```python
from build123d import *

# Parameters (mm, degrees)
SKETCH2_W           = 35
SKETCH2_H           = 35
SKETCH2_R           = 1.6
BOSS_EXTRUDE1_DEPTH = 5
BOSS_EXTRUDE2_DEPTH = 2
SKETCH4_R           = 1.55
BOSS_EXTRUDE3_DEPTH = 2
CUT_EXTRUDE1_DEPTH  = 52.27194652
FILLET1_R           = 2


with BuildPart() as part:
    # Sketch2 → Boss-Extrude1 (new body)
    with BuildSketch(Plane(origin=(0, 0, 0), x_dir=(1, 0, 0), z_dir=(0, 1, 0))):
        Rectangle(SKETCH2_W, SKETCH2_H)
        with Locations(Location((7, 0, 0), (0, 0, 270))):
            Circle(SKETCH2_R, mode=Mode.SUBTRACT)
        with Locations(Location((-3.5, -6.062177826, 0), (0, 0, 270))):
            Circle(SKETCH2_R, mode=Mode.SUBTRACT)
        with Locations(Location((-3.5, 6.062177826, 0), (0, 0, 270))):
            Circle(SKETCH2_R, mode=Mode.SUBTRACT)
    extrude(amount=BOSS_EXTRUDE1_DEPTH)

    # Sketch3 → Boss-Extrude2 (add)
    with BuildSketch(Plane(origin=(17.5, 0, 0), x_dir=(0, 0, -1), z_dir=(1, 0, 0))):
        Polygon((-17.5, 0), (-27.5, 18.75), (17.5, 18.75), (17.5, 0), align=None)
    boss_extrude2 = extrude(amount=BOSS_EXTRUDE2_DEPTH)

    # Mirror1: Boss-Extrude2 across plane
    add(boss_extrude2.mirror(Plane(origin=(0, 0, 0), x_dir=(0, 0, 1), z_dir=(1, 0, 0))))

    # Sketch4 → Boss-Extrude3 (add)
    with BuildSketch(Plane(origin=(0, 18.75, 0), x_dir=(1, 0, 0), z_dir=(0, 1, 0))):
        Polygon((-19.5, -27.5), (-29.5, -27.5), (-19.5, 17.5), align=None)
        with Locations(Location((-23, -22.5, 0), (0, 0, 270))):
            Circle(SKETCH4_R, mode=Mode.SUBTRACT)
        with Locations(Location((-23, -10, 0), (0, 0, 270))):
            Circle(SKETCH4_R, mode=Mode.SUBTRACT)
    boss_extrude3 = extrude(amount=-BOSS_EXTRUDE3_DEPTH)

    # Sketch5 → Cut-Extrude1 (cut, through all)
    with BuildSketch(Plane(origin=(-19.5, 0, 0), x_dir=(0, 0, -1), z_dir=(1, 0, 0))):
        Polygon((-27.5, 18.75), (-26.433333333, 16.75), (-27.5, 16.75), align=None)
    cut_extrude1 = extrude(amount=-CUT_EXTRUDE1_DEPTH, mode=Mode.SUBTRACT)

    # Mirror2: Boss-Extrude3, Cut-Extrude1 across plane
    add(boss_extrude3.mirror(Plane(origin=(0, 0, 0), x_dir=(0, 0, 1), z_dir=(1, 0, 0))))
    add(cut_extrude1.mirror(Plane(origin=(0, 0, 0), x_dir=(0, 0, 1), z_dir=(1, 0, 0))), mode=Mode.SUBTRACT)

    # Fillet1
    fillet1_edges = [part.edges().sort_by_distance(p)[0] for p in [
        (17.5, 11.875, -17.5),
        (-17.5, 11.875, -17.5),
        (-17.5, 18.75, 5),
        (17.5, 18.75, 5),
        (0, 5, -17.5),
        (0, 0, -17.5),
        (17.5, 5, 0),
        (-17.5, 5, 0),
        (-19.5, 0, 0),
        (19.5, 0, 0),
    ]]
    fillet(fillet1_edges, radius=FILLET1_R - 0.0001)  # a hair under: the kernel refuses the full size


solid = part.part
```
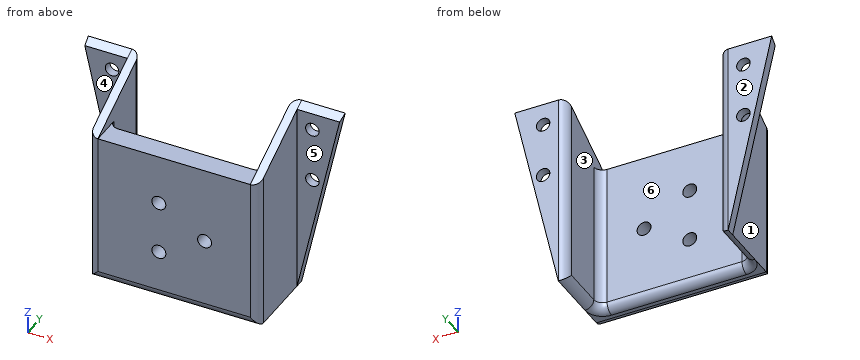
CAD build for the part. Positions are in the model's coordinates, mm. Face numbers are marked on the shaded views. A direction names the side the tool comes from. Round coordinates to 2 decimals unless told otherwise and drop trailing zeros. Order: outer loops, then holes, each group sorted by start corner. A loop starts at its lowest first (then second) coordinate and runs counter-clockwise, first axis right, second up. Notation, with made-up numbers: (47, 3) - (87, 3) arc R10 ccw to (87, 16) - close; hole circle Ø2 at (58, 83). An arc over 180 degrees is marked (long way). Answer as CSV lines item,"result". Start each with the question number.
1. Saw through at B-B, the plane x = -3.5. Write the cut outline in (y, z).
2. Saw through at A-A, the plane x = 7. Write the cut outline in (y, z).
3. Drill centre lines: L1, parallel to X at y = 15.25, z = 23.5; L2, parallel to X at y = 17.6, z = 10; L3, parallel to X at y = 18.2, z = 10. Where is each one in solid material? Low to high. Write a range as [from, to].
4. Pin check, flat tips, straight feed: pin 1 (1.5 mm diameter, centred on y = 5.5, z = 19, fed in from +X); pin 2 (4 mm diameter, centred on x = 8, z = 17.5, fed in from -Y); pin 3 (6 mm diameter, centred on x = 5, z = 9.5, fed in from +Y); pin 4 (5 mm diameter, centred on y = 10.5, z = 7, fed in from -X). Stop position of each tip, or through.
5. Tool access for the marked faces 4, 5 and 6: list every direction of +Z, -Z, +X, -X, +Y, -Y with a clear straight run to the whole face (end or side of a thin tool).
6. Pull direction X, two halves, no side cores. Call the marked faces 1, 2 and 3: +X half, -X half, draft (parallel to the pull), parting line (faces both ways), or undercut.
7. Saw through at C-C, the plane z = 0. Write the cut outline in (x, y), and give its area (3 significant figures).
Model answer:
1,outline,"(0, -15.5) arc R2 ccw to (2, -17.5) - (3, -17.5) arc R2 ccw to (5, -15.5) - (5, -7.66) - (0, -7.66) - close; (0, -4.46) - (5, -4.46) - (5, 4.46) - (0, 4.46) - close; (0, 7.66) - (5, 7.66) - (5, 17.5) - (0, 17.5) - close"
2,outline,"(0, -15.5) arc R2 ccw to (2, -17.5) - (3, -17.5) arc R2 ccw to (5, -15.5) - (5, -1.6) - (0, -1.6) - close; (0, 1.6) - (5, 1.6) - (5, 17.5) - (0, 17.5) - close"
3,L1,"x = [-19.5, -17.5], [17.5, 19.5]"
3,L2,"x = [-25.61, -24.55], [-21.45, -17.69], [17.69, 21.45], [24.55, 25.61]"
3,L3,"x = [-25.61, -24.55], [-21.45, -18.12], [18.12, 21.45], [24.55, 25.61]"
4,pin 1,"stops at x = 19.5"
4,pin 2,"stops at y = 0"
4,pin 3,"stops at y = 5"
4,pin 4,"stops at x = -19.5"
5,face 4,"+Z, -Z, -X, -Y"
5,face 5,"+Z, -Z, +X, -Y"
5,face 6,"+Z, -Z, +Y"
6,face 1,"-X half"
6,face 2,"draft"
6,face 3,"undercut"
7,outline,"(-23.39, 16.75) - (-19.5, 16.75) - (-19.5, 2) arc R2 ccw to (-17.5, 0) - (5.4, 0) - (5.4, 5) - (-15.5, 5) arc R2 cw to (-17.5, 7) - (-17.5, 16.75) arc R2 ccw to (-19.5, 18.75) - (-23.39, 18.75) - close; (8.6, 0) - (17.5, 0) arc R2 ccw to (19.5, 2) - (19.5, 16.75) - (23.39, 16.75) - (23.39, 18.75) - (19.5, 18.75) arc R2 ccw to (17.5, 16.75) - (17.5, 7) arc R2 cw to (15.5, 5) - (8.6, 5) - close"
7,area,"248 mm²"
